Part model, mm, in its own coordinate system. A direction names the side the tool comes from. Give positions to 0.01 mm unless a question says otherwise; leave off trailing zeros. Order: outer loops, then holes, each group sorted by start corner. A loop starts at its lowest first (then second) coordinate and runs counter-clockwise, first axis right, second up.
from build123d import *

# Parameters (mm, degrees)
CROQUIS1_R              = 7.5
CROQUIS1_R_2            = 2
CROQUIS1_W              = 3
CROQUIS1_H              = 28
SALIENTE_EXTRUIR1_DEPTH = 100
CROQUIS2_R              = 7.5
SALIENTE_EXTRUIR2_DEPTH = 115
CROQUIS3_R              = 2
CORTAR_EXTRUIR2_DEPTH   = 149
CROQUIS4_R              = 2
SALIENTE_EXTRUIR3_DEPTH = 86
CROQUIS5_R              = 2
CORTAR_EXTRUIR3_DEPTH   = 139
CROQUIS7_R              = 2
CORTAR_EXTRUIR4_DEPTH   = 139
CROQUIS8_R              = 2
SALIENTE_EXTRUIR4_DEPTH = 78
CROQUIS9_R              = 2
CORTAR_EXTRUIR5_DEPTH   = 117


with BuildPart() as part:
    # Croquis1 → Saliente-Extruir1 (new body)
    with BuildSketch(Plane(origin=(0, 0, 0), x_dir=(1, 0, 0), z_dir=(0, 1, 0))):
        with BuildLine():
            Line((0, 0), (0, 40))
            Line((0, 40), (80, 40))
            Line((80, 40), (80, 0))
            Line((80, 0), (100, 0))
            Line((100, 0), (100, 40))
            Line((100, 40), (180, 40))
            Line((180, 40), (180, 0))
            Line((180, 0), (195, 0))
            ThreePointArc((195, 0), (202.071067812, 2.928932188), (205, 10))
            Line((205, 10), (205, 190))
            ThreePointArc((205, 190), (202.071067812, 197.071067812), (195, 200))
            Line((195, 200), (180, 200))
            Line((180, 200), (180, 160))
            Line((180, 160), (100, 160))
            Line((100, 160), (100, 200))
            Line((100, 200), (80, 200))
            Line((80, 200), (80, 160))
            Line((80, 160), (0, 160))
            Line((0, 160), (0, 200))
            Line((0, 200), (-5, 200))
            ThreePointArc((-5, 200), (-19.142135624, 194.142135624), (-25, 180))
            Line((-25, 180), (-25, 20))
            ThreePointArc((-25, 20), (-19.142135624, 5.857864376), (-5, 0))
            Line((-5, 0), (0, 0))
        make_face()
        with Locations(Location((-5, 70, 0), (0, 0, 270))):
            Circle(CROQUIS1_R, mode=Mode.SUBTRACT)
        with Locations(Location((-5, 130, 0), (0, 0, 270))):
            Circle(CROQUIS1_R, mode=Mode.SUBTRACT)
        with Locations(Location((192.5, 170, 0), (0, 0, 270))):
            Circle(CROQUIS1_R, mode=Mode.SUBTRACT)
        with Locations(Location((192.5, 30, 0), (0, 0, 270))):
            Circle(CROQUIS1_R, mode=Mode.SUBTRACT)
        with Locations(Location((90, 98.617815675, 0), (0, 0, 270))):
            Circle(CROQUIS1_R, mode=Mode.SUBTRACT)
        with Locations(Location((32.5, 152, 0), (0, 0, 270))):
            Circle(CROQUIS1_R_2, mode=Mode.SUBTRACT)
        with Locations(Location((47.5, 152, 0), (0, 0, 270))):
            Circle(CROQUIS1_R_2, mode=Mode.SUBTRACT)
        with Locations(Location((47.5, 137, 0), (0, 0, 270))):
            Circle(CROQUIS1_R_2, mode=Mode.SUBTRACT)
        with Locations(Location((32.5, 137, 0), (0, 0, 270))):
            Circle(CROQUIS1_R_2, mode=Mode.SUBTRACT)
        with Locations(Location((32.5, 48, 0), (0, 0, 270))):
            Circle(CROQUIS1_R_2, mode=Mode.SUBTRACT)
        with Locations(Location((32.5, 63, 0), (0, 0, 270))):
            Circle(CROQUIS1_R_2, mode=Mode.SUBTRACT)
        with Locations(Location((47.5, 48, 0), (0, 0, 270))):
            Circle(CROQUIS1_R_2, mode=Mode.SUBTRACT)
        with Locations(Location((47.5, 63, 0), (0, 0, 270))):
            Circle(CROQUIS1_R_2, mode=Mode.SUBTRACT)
        with Locations(Location((132.5, 152, 0), (0, 0, 270))):
            Circle(CROQUIS1_R_2, mode=Mode.SUBTRACT)
        with Locations(Location((132.5, 137, 0), (0, 0, 270))):
            Circle(CROQUIS1_R_2, mode=Mode.SUBTRACT)
        with Locations(Location((147.5, 152, 0), (0, 0, 270))):
            Circle(CROQUIS1_R_2, mode=Mode.SUBTRACT)
        with Locations(Location((147.5, 137, 0), (0, 0, 270))):
            Circle(CROQUIS1_R_2, mode=Mode.SUBTRACT)
        with Locations(Location((132.5, 63, 0), (0, 0, 270))):
            Circle(CROQUIS1_R_2, mode=Mode.SUBTRACT)
        with Locations(Location((132.5, 48, 0), (0, 0, 270))):
            Circle(CROQUIS1_R_2, mode=Mode.SUBTRACT)
        with Locations(Location((147.5, 63, 0), (0, 0, 270))):
            Circle(CROQUIS1_R_2, mode=Mode.SUBTRACT)
        with Locations(Location((147.5, 48, 0), (0, 0, 270))):
            Circle(CROQUIS1_R_2, mode=Mode.SUBTRACT)
        with Locations(Location((90, 50, 0), (0, 0, 270))):
            Circle(CROQUIS1_R_2, mode=Mode.SUBTRACT)
        with Locations(Location((185, 50, 0), (0, 0, 270))):
            Circle(CROQUIS1_R_2, mode=Mode.SUBTRACT)
        with Locations(Location((185, 150, 0), (0, 0, 270))):
            Circle(CROQUIS1_R_2, mode=Mode.SUBTRACT)
        with Locations(Location((90, 150, 0), (0, 0, 270))):
            Circle(CROQUIS1_R_2, mode=Mode.SUBTRACT)
        with Locations((-8.5, 99.450016357)):
            Rectangle(CROQUIS1_W, CROQUIS1_H, mode=Mode.SUBTRACT)
    extrude(amount=-SALIENTE_EXTRUIR1_DEPTH)

    # Croquis2 → Saliente-Extruir2 (add)
    with BuildSketch(Plane(origin=(0, 0, 0), x_dir=(1, 0, 0), z_dir=(0, 1, 0))):
        with Locations(Location((-5, 130, 0), (0, 0, 270))):
            Circle(CROQUIS2_R)
        with Locations(Location((-5, 70, 0), (0, 0, 270))):
            Circle(CROQUIS2_R)
    extrude(amount=-SALIENTE_EXTRUIR2_DEPTH)

    # Croquis3 → Cortar-Extruir2 (cut)
    with BuildSketch(Plane(origin=(0, 0, 0), x_dir=(1, 0, 0), z_dir=(0, 1, 0))):
        with Locations(Location((-11, 117.450016357, 0), (0, 0, 270))):
            Circle(CROQUIS3_R)
        with Locations(Location((-11, 81.450016357, 0), (0, 0, 270))):
            Circle(CROQUIS3_R)
        with Locations(Location((190, 76, 0), (0, 0, 270))):
            Circle(CROQUIS3_R)
        with Locations(Location((-12.5, 25.729751891, 0), (0, 0, 270))):
            Circle(CROQUIS3_R)
        with Locations(Location((-12.5, 10.729751891, 0), (0, 0, 270))):
            Circle(CROQUIS3_R)
        with Locations(Location((190, 124, 0), (0, 0, 270))):
            Circle(CROQUIS3_R)
        with Locations(Location((93, 124, 0), (0, 0, 270))):
            Circle(CROQUIS3_R)
        with Locations(Location((100, 76, 0), (0, 0, 270))):
            Circle(CROQUIS3_R)
    extrude(amount=-CORTAR_EXTRUIR2_DEPTH, mode=Mode.SUBTRACT)

    # Croquis4 → Saliente-Extruir3 (add)
    with BuildSketch(Plane(origin=(0, 0, 0), x_dir=(1, 0, 0), z_dir=(0, 1, 0))):
        with Locations(Location((-12.5, 25.729751891, 0), (0, 0, 270))):
            Circle(CROQUIS4_R)
        with Locations(Location((-12.5, 10.729751891, 0), (0, 0, 270))):
            Circle(CROQUIS4_R)
    extrude(amount=-SALIENTE_EXTRUIR3_DEPTH)

    # Croquis5 → Cortar-Extruir3 (cut)
    with BuildSketch(Plane(origin=(0, 0, 0), x_dir=(1, 0, 0), z_dir=(0, 1, 0))):
        with Locations(Location((-11, 40, 0), (0, 0, 270))):
            Circle(CROQUIS5_R)
        with Locations(Location((-11, 25, 0), (0, 0, 270))):
            Circle(CROQUIS5_R)
    extrude(amount=-CORTAR_EXTRUIR3_DEPTH, mode=Mode.SUBTRACT)

    # Croquis7 → Cortar-Extruir4 (cut)
    with BuildSketch(Plane(origin=(0, 0, 0), x_dir=(1, 0, 0), z_dir=(0, 1, 0))):
        with Locations(Location((-11, 145, 0), (0, 0, 270))):
            Circle(CROQUIS7_R)
        with Locations(Location((-11, 55, 0), (0, 0, 270))):
            Circle(CROQUIS7_R)
    extrude(amount=-CORTAR_EXTRUIR4_DEPTH, mode=Mode.SUBTRACT)

    # Croquis8 → Saliente-Extruir4 (add)
    with BuildSketch(Plane(origin=(0, 0, 0), x_dir=(1, 0, 0), z_dir=(0, 1, 0))):
        with Locations(Location((-11, 40, 0), (0, 0, 270))):
            Circle(CROQUIS8_R)
        with Locations(Location((-11, 25, 0), (0, 0, 270))):
            Circle(CROQUIS8_R)
    extrude(amount=-SALIENTE_EXTRUIR4_DEPTH)

    # Croquis9 → Cortar-Extruir5 (cut)
    with BuildSketch(Plane(origin=(0, 0, 0), x_dir=(1, 0, 0), z_dir=(0, 1, 0))):
        with Locations(Location((-11, 27.5, 0), (0, 0, 270))):
            Circle(CROQUIS9_R)
        with Locations(Location((-11, 12.5, 0), (0, 0, 270))):
            Circle(CROQUIS9_R)
    extrude(amount=-CORTAR_EXTRUIR5_DEPTH, mode=Mode.SUBTRACT)


solid = part.part
Item 1: Band-saw the part on A-A on z = -186.5. List the corners of the cut face in (x, y).
Item 2: Drill centre lines: probe 1 along X at (y, z) = (-40, -63); probe 2 along X at (y, z) = (-60, -13) (1 decimal); probe 3 along Z at (x, y) = (49, -10.5). Where is each one in solid material? Low to high.
Item 3: Band-saw the part on D-D on x = 139. List the corners of the cut face in (y, z), plus the area to 3 significant figures.
Item 4: Pull direction Z, two halves, no side cores. Call faces 6 (the face through (100, -49, -20)), 7 (the face through (-18.986, -49.3, -194.297)), 8 (the face through (199.936, -49.3, -30.976)): released by +Z, released by -Z, zero draft, split by the parting line, or undercut.
Item 5: Drop flat-ended pins along their axis: P1, Ø12, axis at x = 68.5, y = -78.5, coming from the +Z side; P2, Ø0.9, axis at x = -8, y = -45.5, coming from the +Z side; P3, Ø3, axis at x = 147.5, z = -63, coming from the +Y side; P4, Ø6, axis at x = 22, y = -20.5, coming from the -Z side. Give the stop position or say it passes through.
Item 6: Band-saw the part on C-C on z = -70. List the corners of the cut face in (x, y).
Item 7: Band-saw the part on B-B on y = -65. Give the number of separate pieces and of enclosed holes in the cut face, plus the area to 3 significant figures.
Item 8: Which spindle directions (+Z, -Z, +X, -X, +Y, -Y) get a long thin tool onto all of the face, cutting with end or side? Do faces 1 (the face through (141, -49, -160)), 2 (the face through (90, -49, 0)), 3 (the face through (-2.747, -107.395, -122.846)), 4 (the face through (180, -49, -20)), 5 (the face through (117, 0, -101)). Say none if no direction does.
Working result:
1. outline: (-23.91, -100) - (0, -100) - (0, 0) - (-23.91, 0) - close; (80, -100) - (100, -100) - (100, 0) - (80, 0) - close; (180, -100) - (205, -100) - (205, 0) - (180, 0) - close
2. probe 1: x = -25 to 30.5, 34.5 to 45.5, 49.5 to 130.5, 134.5 to 145.5, 149.5 to 205
2. probe 2: x = -23.7 to -12.9, -9.1 to 0, 80 to 100, 180 to 205
2. probe 3: z = -160 to -153.32, -150.68 to -138.32, -135.68 to -64.32, -61.68 to -49.32, -46.68 to -40
3. outline: (-100, -160) - (0, -160) - (0, -40) - (-100, -40) - close
3. area: 12,000 mm2
4. face 6: zero draft
4. face 7: released by -Z
4. face 8: undercut
5. P1: stops at z = -40
5. P2: stops at z = -0.16
5. P3: passes through
5. P4: stops at z = -160
6. outline: (-25, -100) - (-12.5, -100) - (-12.5, -115) - (2.5, -115) - (2.5, -100) - (205, -100) - (205, 0) - (-25, 0) - close
7. separate pieces: 1
7. enclosed holes: 34
7. area: 32,000 mm2
8. face 1: -Z, +Y, -Y
8. face 2: +Z, +X, -X, +Y, -Y
8. face 3: -Y
8. face 4: +Z, +Y, -Y
8. face 5: +Z, -Z, +X, -X, +Y
